```python
from build123d import *

# Parameters (mm, degrees)
EXTRUDE_2_DEPTH      = 0.95
EXTRUDE_2_DEPTH_BACK = 0.95
FILLET_6_R           = 8
CHAMFER_1_SIZE       = 0.5
CHAMFER_2_SIZE       = 0.5
CHAMFER_2_SIZE2      = 0.436431784


with BuildPart() as part:
    # 草图3 → 凸台-拉伸2 (new, two sides: drawn at the far end of the back side and taken through both)
    with BuildSketch(Plane(origin=(0, 0, 0), x_dir=(1, 0, 0), z_dir=(0, 1, 0)).offset(-EXTRUDE_2_DEPTH_BACK)):
        Polygon((-187.120164296, -75.485656639), (-188.025009302, -71.812776929), (-195.252497915, -74.872539862), (-199.736508362, -82.868381819), (-198.907982221, -83.333013297), (-206.244927345, -96.416179437), (-205.305528647, -96.942987446), (-212.153344095, -109.15394251), (-211.528903604, -109.50412423), (-217.926627044, -120.91247979), (-218.646393726, -127.274440762), (-218.168094082, -127.536139913), (-190.089143959, -76.21708991), align=None)
    extrude(amount=EXTRUDE_2_DEPTH + EXTRUDE_2_DEPTH_BACK)

    # 圆角6
    fillet_6_edges = [part.edges().sort_by_distance(p)[0] for p in [
        (-195.252497915, 0, 74.872539862),
    ]]
    fillet(fillet_6_edges, radius=FILLET_6_R)

    # 倒角1
    chamfer_1_edges = [part.edges().sort_by_distance(p)[0] for p in [
        (-187.120164296, 0, 75.485656639),
    ]]
    chamfer(chamfer_1_edges, length=CHAMFER_1_SIZE)

    # 倒角2
    chamfer_2_edges = [part.edges().sort_by_distance(p)[0] for p in [
        (-188.025009302, 0, 71.812776929),
    ]]
    chamfer_2_side = [part.faces().sort_by_distance(p)[0] for p in [
        (-190.378641555, 0, 72.809188977),
    ]]
    chamfer(chamfer_2_edges, length=CHAMFER_2_SIZE, length2=CHAMFER_2_SIZE2, reference=chamfer_2_side[0])


solid = part.part
```
Input: part model. Units: mm. Frame: model coordinates. Give positions to 0.01 mm unless a question says otherwise; leave off trailing zeros. Write each loop counter-clockwise with the first axis right and the second up, starting at its lowest first coordinate (ties: lowest second). Pieces come first, ordered by that corner, then holes. Notation, with made-up numbers: (7.25, 54.25) - (21.25, 54.25) arc R27 ccw to (21.25, 74.25) - close; hole circle Ø4 at (70.5, 60.5). An arc over 180 degrees is marked (long way). Write item = value, one per line. Start each with the question number.
1) Cut plane B-B (z = 99.5). Return loops of the section in (x, y).
2) Material intervals for L1, parallel to Z at x = -206, y = -0.7; L2, parallel to X at y = -0.75, z = 99.5; L3, parallel to Z at x = -192, y = -0.15, sorted ascending. Write a range as [from, to].
3) Pin query (flat end, axial travel): pin 1 (1 mm diameter, centred on y = 0.5, z = 79.5, fed in from -X). Return the tip coordinate at first contact, or that it passes through.
4) Cut plane A-A (y = 0.2). Return loops of the section in (x, z), and give its area (3 significant figures).
5) Cut plane C-C (x = -201.5). Return loops of the section in (y, z), and give its area (3 significant figures).
Answers follow:
q1.outline = (-206.74, -0.95) - (-202.83, -0.95) - (-202.83, 0.95) - (-206.74, 0.95) - close
q2.L1 = [95.98, 96.55], [98.18, 105.3]
q2.L2 = [-206.74, -202.83]
q2.L3 = [73.5, 79.71]
q3.pin_1 = -198.13
q4.outline = (-218.65, 127.27) - (-217.93, 120.91) - (-211.53, 109.5) - (-212.15, 109.15) - (-205.31, 96.94) - (-206.24, 96.42) - (-198.91, 83.33) - (-199.74, 82.87) - (-196.59, 77.26) arc R8 ccw to (-192.73, 73.81) - (-188.49, 72.01) - (-187.92, 72.24) - (-187.24, 75) - (-187.61, 75.61) - (-190.09, 76.22) - (-218.17, 127.54) - close
q4.area = 232 mm^2
q5.outline = (-0.95, 87.96) - (0.95, 87.96) - (0.95, 97.07) - (-0.95, 97.07) - close
q5.area = 17.3 mm^2
